Design review of the part built by this model. Coordinates are the model's own, in mm. Face numbers are marked on the shaded views. Round coordinates to 2 decimals unless told otherwise and drop trailing zeros. Loops run counter-clockwise (first coordinate to the right, second up) from the corner with the lowest first, then second, coordinate; pieces in that order, holes last. Notation, with made-up numbers: (5, -20) - (54, -20) arc R16 ccw to (54, -14) - close; hole circle Ø2 at (75, -4.5). An arc over 180 degrees is marked (long way). Return JSON: item names as keys, results as strings. Group by question number.
(1) We need section B-B, the plane x = 0. Write out the cut boundary in (y, z), and give its area (3 significant figures).
(2) We need section D-D, the plane x = 23. Write out the cut boundary in (y, z).
(3) We need section A-A, the plane z = 0. Write out the cut boundary in (x, y).
(4) We need section C-C, the plane y = -10. Write out the cut boundary in (x, z), and give its area (3 significant figures).
(5) Clearance check with flat-ended pins moving along their axes: pin 1 (17.5 mm diameter, centred on x = 24.55, z = -24.55, fed in from -Y); pin 2 (2 mm diameter, centred on y = -6, z = -28, fed in from -X); pin 3 (2 mm diameter, centred on y = -8, z = -15, fed in from +X). State where each tip first meets the part, or that it passes through.
(6) Wall thickness on L1, parallel to Z at x = 0, y = -1.5; L2, parallel to X at y = -2.5, z = -1.5; L3, parallel to X at y = -0.75, z = -24: over which ranges is each line inside the solid? List them lowest first. Write a range as [from, to].
(7) The part is to be moulded in two halves that separate along X. For the marked faces 1 and 2, say which applies: pulls with the +X half, pulls with the -X half, needs draft (parallel to the pull), parting line crosses it, or undercut.
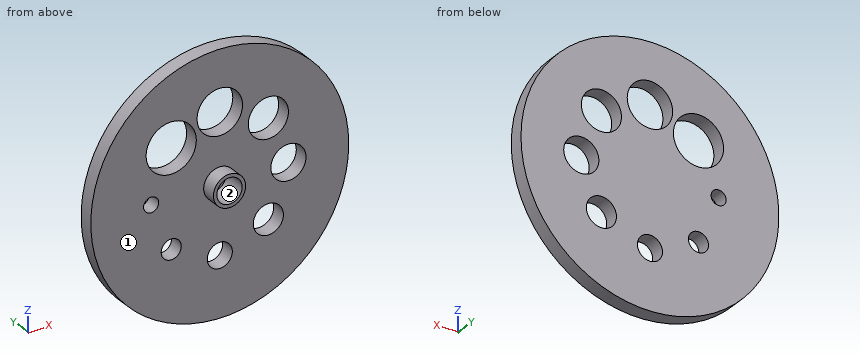
from build123d import *

# Parameters (mm, degrees)
F0_R      = 65.21802
F0_R_2    = 5.08
F0_R_3    = 6.35
F0_R_4    = 7.62
F0_R_5    = 3.81
F0_R_6    = 12.6873
F0_R_7    = 10.16
F0_R_8    = 8.89
F0_R_9    = 11.4935
F1_DEPTH  = 7.62
F2_R      = 8.138999
F2_R_2    = 6.4008
F3_DEPTH  = 15.24
F3_FACE_R = 6.4008
F4_DEPTH  = 5.08


with BuildPart() as f1:
    # F0 (on Front) → F1 (new body)
    with BuildSketch(Plane.XZ):
        Circle(F0_R)
        with Locations((-24.55202, -24.55202)):
            Circle(F0_R_2, mode=Mode.SUBTRACT)
        with Locations((0, -34.7218)):
            Circle(F0_R_3, mode=Mode.SUBTRACT)
        with Locations((24.55202, -24.55202)):
            Circle(F0_R_4, mode=Mode.SUBTRACT)
        with Locations((-34.7218, 0)):
            Circle(F0_R_5, mode=Mode.SUBTRACT)
        with Locations((-24.55202, 24.55202)):
            Circle(F0_R_6, mode=Mode.SUBTRACT)
        with Locations((24.55202, 24.55202)):
            Circle(F0_R_7, mode=Mode.SUBTRACT)
        with Locations((34.7218, 0)):
            Circle(F0_R_8, mode=Mode.SUBTRACT)
        with Locations((0, 34.7218)):
            Circle(F0_R_9, mode=Mode.SUBTRACT)
    extrude(amount=F1_DEPTH)

    # F2 (on Front) → F3 (join)
    with BuildSketch(Plane.XZ):
        Circle(F2_R)
        Circle(F2_R_2, mode=Mode.SUBTRACT)
    extrude(amount=F3_DEPTH)

    # F3_face (on face) → F4 (cut)
    with BuildSketch(Plane.XZ.offset(7.62)):
        Circle(F3_FACE_R)
    extrude(amount=-F4_DEPTH, mode=Mode.SUBTRACT)


solid = f1.part
Solutions:
{
 "1": {"outline": "(-15.24, -8.14) - (-7.62, -8.14) - (-7.62, -28.37) - (0, -28.37) - (0, 23.23) - (-7.62, 23.23) - (-7.62, 8.14) - (-15.24, 8.14) - (-15.24, 6.4) - (-2.54, 6.4) - (-2.54, -6.4) - (-15.24, -6.4) - close; (-7.62, -65.22) - (0, -65.22) - (0, -41.07) - (-7.62, -41.07) - close; (-7.62, 46.22) - (0, 46.22) - (0, 65.22) - (-7.62, 65.22) - close", "area": "683 mm^2"},
 "2": {"outline": "(-7.62, -61.03) - (0, -61.03) - (0, -32.01) - (-7.62, -32.01) - close; (-7.62, -17.09) - (0, -17.09) - (0, 14.51) - (-7.62, 14.51) - close; (-7.62, 34.59) - (0, 34.59) - (0, 61.03) - (-7.62, 61.03) - close"},
 "3": {"outline": "(-65.22, -7.62) - (-38.53, -7.62) - (-38.53, 0) - (-65.22, 0) - close; (-30.91, -7.62) - (-8.14, -7.62) - (-8.14, -15.24) - (-6.4, -15.24) - (-6.4, -2.54) - (6.4, -2.54) - (6.4, -15.24) - (8.14, -15.24) - (8.14, -7.62) - (25.83, -7.62) - (25.83, 0) - (-30.91, 0) - close; (43.61, -7.62) - (65.22, -7.62) - (65.22, 0) - (43.61, 0) - close"},
 "4": {"outline": "circle Ø16.28 at (0, 0); hole circle Ø12.8 at (0, 0)", "area": "79.4 mm^2"},
 "5": {"pin 1": "y = -7.62", "pin 2": "x = -59.37", "pin 3": "x = 63.68"},
 "6": {"L1": "[-65.22, -41.07], [-28.37, 23.23], [46.22, 65.22]", "L2": "[-65.2, -38.22], [-31.22, 25.96], [43.48, 65.2]", "L3": "[-60.64, -29.6], [-19.5, 16.95], [32.15, 60.64]"},
 "7": {"face 1": "needs draft", "face 2": "undercut"}
}
